Design review of the part built by this model. Coordinates are the model's own, in mm. A direction names the side the tool comes from. Coordinates: 2 decimals unless noted, no trailing zeros. Write each loop counter-clockwise with the first axis right and the second up, starting at its lowest first coordinate (ties: lowest second). Pieces come first, ordered by that corner, then holes.
Q1. Take a section at C-C, the plane x = 45.48. Write out the cut boundary in (y, z).
Q2. For L1, parallel to Z at x = 6, y = 1.85; L2, parallel to Z at x = 9, y = 1.05; L3, parallel to Z at x = 30.5, y = 1, list the stretches that pass through material, from the lowest coordinate up.
Q3. Take a section at D-D, the plane z = 7. Write out the cut boundary in (x, y).
Q4. Take a section at A-A, the plane x = 33. Write out the cut boundary in (y, z).
Q5. For faces 4 (the flat face through (22, 1, -49.413)), 5 (the flat face through (0, 1, -43)), 6 (the flat face through (10, 1, -39.701)), 7 (the cylindrical face through (50.57, 0.99, -45.59)), 8 (the flat face through (16, 1, -36.692)), list the 3-axis set-ups (+Z, -Z, +X, -X, +Y, -Y) from which the entire face can be reached by the end or side of a thin tool; tool diameter is ignored.
Q6. The part is to be moulded in two halves that separate along X. For faces 1 (the flat face through (41.3, 2, -15.2)), 2 (the cylindrical face through (53.076, 0.986, -8.592)), 3 (the cylindrical face through (44.263, 0.986, -43.288)), say which applies: released by +X, released by -X, zero draft, split by the parting line, or undercut.
Q7. Take a section at B-B, the plane y = 1.5. Write out the cut boundary in (x, z).
Q8. For pin 1 Ø1 at (y, z) = (1, -21) entering from -X; pin 2 Ø5 at (x, z) = (45.48, -41.7) entering from -Y, all flat-tipped, find the tip position at first contact; note any pin that passes through.
from build123d import *

# Parameters (mm, degrees)
SKETCH1_R           = 2
BOSS_EXTRUDE2_DEPTH = 2
FILLET1_R           = 1
FILLET2_R           = 1


with BuildPart() as part:
    # Sketch1 → Boss-Extrude2 (new body)
    with BuildSketch(Plane(origin=(0, 0, 0), x_dir=(1, 0, 0), z_dir=(0, 1, 0))):
        with BuildLine():
            Line((0, 48.412862342), (0, 37.692030173))
            ThreePointArc((0, 37.692030173), (0.292893219, 36.984923392), (1, 36.692030173))
            Line((1, 36.692030173), (31.48, 36.692030173))
            ThreePointArc((31.48, 36.692030173), (38.551067812, 33.763097985), (41.48, 26.692030173))
            Line((41.48, 26.692030173), (41.48, 17.837278162))
            ThreePointArc((41.48, 17.837278162), (40.75973427, 14.11081444), (38.702693625, 10.92115954))
            Line((38.702693625, 10.92115954), (-9.52, -39.4391308))
            Line((-9.52, -39.4391308), (-9.52, -49.4391308))
            Line((-9.52, -49.4391308), (50.011362769, 4.385719046))
            ThreePointArc((50.011362769, 4.385719046), (53.106383896, 8.659526457), (54.200832168, 13.821577266))
            Line((54.200832168, 13.821577266), (54.200832168, 36.692030173))
            ThreePointArc((54.200832168, 36.692030173), (50.474986688, 45.687016862), (41.48, 49.412862342))
            Line((41.48, 49.412862342), (1, 49.412862342))
            ThreePointArc((1, 49.412862342), (0.292893219, 49.119969123), (0, 48.412862342))
        make_face()
        with Locations(Location((45.48, 41.700609081, 0), (0, 0, 270))):
            Circle(SKETCH1_R, mode=Mode.SUBTRACT)
        with BuildLine():
            Line((15, 43.700609081), (4.549516448, 43.700609081))
            Line((4.549516448, 43.700609081), (4.549516448, 39.700609081))
            Line((4.549516448, 39.700609081), (15, 39.700609081))
            ThreePointArc((15, 39.700609081), (17, 41.700609081), (15, 43.700609081))
        make_face(mode=Mode.SUBTRACT)
    extrude(amount=BOSS_EXTRUDE2_DEPTH)

    # Fillet1
    fillet1_edges = [part.edges().sort_by_distance(p)[0] for p in [
        (-9.52, 2, 44.4391308),
    ]]
    fillet(fillet1_edges, radius=FILLET1_R)

    # Fillet2
    fillet2_edges = [part.edges().sort_by_distance(p)[0] for p in [
        (-9.52, 0, 44.4391308),
    ]]
    fillet(fillet2_edges, radius=FILLET2_R - 0.0001)  # a hair under: the kernel refuses the full size


solid = part.part
Responses:
1. outline: (0, -48.77) - (2, -48.77) - (2, -43.7) - (0, -43.7) - close; (0, -39.7) - (2, -39.7) - (2, -0.29) - (0, -0.29) - close
2. L1: z = -49.41 to -43.7, -39.7 to -36.69, 23.23 to 35.41
2. L2: z = -49.41 to -43.7, -39.7 to -36.69, 20.1 to 32.69
2. L3: z = -49.41 to -36.69, -2.35 to 13.26
3. outline: (21.54, 0) - (37.42, 0) - (37.42, 2) - (21.54, 2) - close
4. outline: (0, -49.41) - (2, -49.41) - (2, -36.58) - (0, -36.58) - close; (0, -4.97) - (2, -4.97) - (2, 10.99) - (0, 10.99) - close
5. face 4: -Z, +X, -X, +Y, -Y
5. face 5: -Z, -X, +Y, -Y
5. face 6: +Y, -Y
5. face 7: -Z, +X, +Y, -Y
5. face 8: -X, +Y, -Y
6. face 1: zero draft
6. face 2: released by +X
6. face 3: undercut
7. outline: (-9.39, 39.3) - (38.7, -10.92) arc R10 cw to (41.48, -17.84) - (41.48, -26.69) arc R10 cw to (31.48, -36.69) - (1, -36.69) arc R1 ccw to (0, -37.69) - (0, -48.41) arc R1 ccw to (1, -49.41) - (41.48, -49.41) arc R12.72 ccw to (54.2, -36.69) - (54.2, -13.82) arc R12.72 ccw to (50.01, -4.39) - (-9.39, 49.32) - close; hole (4.55, -43.7) - (15, -43.7) arc R2 ccw to (15, -39.7) - (4.55, -39.7) - close; hole circle Ø4 at (45.48, -41.7)
8. pin 1: stops at x = 41.48
8. pin 2: stops at y = 0
